from build123d import *

# Parameters (mm, degrees)
EXTRUDE1_DEPTH = 76.968
EXTRUDE2_DEPTH = 90
EXTRUDE3_DEPTH = 101.968
EXTRUDE4_DEPTH = 76.321
EXTRUDE5_DEPTH = 126.968
EXTRUDE6_DEPTH = 126.968
EXTRUDE7_DEPTH = 88.484


with BuildPart() as part:
    # Sketch1 → Extrude1 (new body)
    with BuildSketch(Plane(origin=(0, 0, 0), x_dir=(1, 0, 0), z_dir=(0, 1, 0))):
        Polygon((0, 0), (0, 55), (90, 77.5), (90, -22.5), align=None)
    extrude(amount=EXTRUDE1_DEPTH)

    # Sketch2 → Extrude2 (cut, symmetric)
    with BuildSketch(Plane.XY):
        Polygon((90, 76.968), (0, 35.000310766), (0, 76.968), align=None)
    extrude(amount=EXTRUDE2_DEPTH, both=True, mode=Mode.SUBTRACT)

    # Sketch3 → Extrude3 (add)
    with BuildSketch(Plane(origin=(0, 0, 0), x_dir=(1, 0, 0), z_dir=(0, 1, 0))):
        Polygon((90, 62.5), (20, 45), (20, 10), (90, -7.5), align=None)
    extrude(amount=EXTRUDE3_DEPTH)

    # Sketch4 → Extrude4 (cut, symmetric)
    with BuildSketch(Plane.XY):
        Polygon((90, 101.968), (20, 69.326463929), (20, 101.968), align=None)
    extrude(amount=EXTRUDE4_DEPTH, both=True, mode=Mode.SUBTRACT)

    # Sketch5 → Extrude5 (add)
    with BuildSketch(Plane(origin=(0, 0, 0), x_dir=(1, 0, 0), z_dir=(0, 1, 0))):
        Polygon((90, 47.5), (40, 35), (40, 20), (90, 7.5), align=None)
    extrude(amount=EXTRUDE5_DEPTH)

    # Sketch6 → Extrude6 (cut)
    with BuildSketch(Plane.XY):
        Polygon((90, 126.968), (40, 103.652617092), (40, 126.968), align=None)
    extrude(amount=-EXTRUDE6_DEPTH, mode=Mode.SUBTRACT)

    # Sketch7 → Extrude7 (cut, symmetric)
    with BuildSketch(Plane.XY):
        with BuildLine():
            Line((80, 0), (10, 0))
            ThreePointArc((10, 0), (45, 35), (80, 0))
        make_face()
    extrude(amount=EXTRUDE7_DEPTH, both=True, mode=Mode.SUBTRACT)


solid = part.part
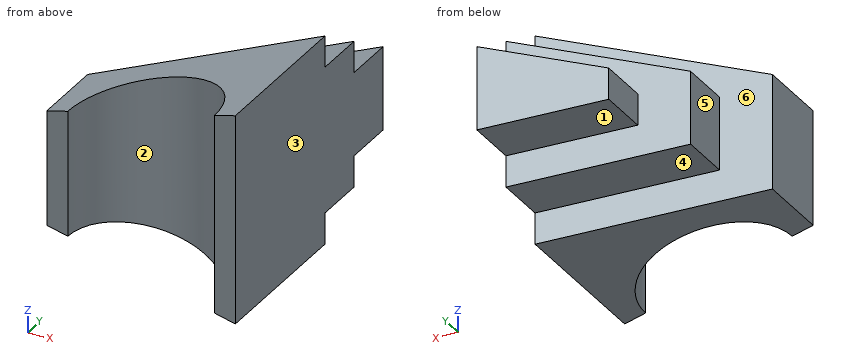
Check sheet for the modelled part. Datum: model origin and axes. Units: mm. Face numbers are marked on the shaded views. A direction names the side the tool comes from. Give positions to 0.01 mm unless a question says otherwise; leave off trailing zeros. Loops run counter-clockwise (first coordinate to the right, second up) from the corner with the lowest first, then second, coordinate; pieces in that order, holes last. Notation, with made-up numbers: M -5,4.25 L 24,4.25 A17 ccw 24,29.25 Z; hole C -24,66 d8. An arc over 180 degrees is marked long. Answer as a JSON object with one key per item and string values. Group by question number.
Q1. Cross-section at C-C on z = -5. Record the cut outline in (x, y), then the cut area to 3 significant figures.
Q2. Cross-section at D-D on y = 87. Record the cut outline in (x, z).
Q3. Release check for a two-part mould opening along X. For the marked faces 1, 2 and 3 record: released by +X, released by -X, zero draft, split by the parting line, or undercut.
Q4. Cross-section at B-B on x = 69. Record the cut outline in (y, z), then the cut area to 3 significant figures.
Q5. Go/stop test with flat-tipped pins: P1, Ø4, axis at y = 41, z = -12.5, coming from the -X side; P2, Ø1, axis at x = 50, z = -45, coming from the +Y side; P3, Ø6, axis at x = 16, z = -65, coming from the +Y side; P4, Ø2, axis at x = 80, y = 63.5, coming from the +Z side. Record where each tip stops, or that it passes through.
Q6. Cross-section at A-A on y = 10.5. Record the cut outline in (x, z), then the cut area to 3 significant figures.
Q7. Access from +Z, -Z, +X, -X, +Y, -Y to the whole of each face (thin tool, end or side, straight path). Record for the marked faces 4, 5 and 6.
Q8. Material ranges on line 1 along X through (y, z) = (95, -31.5); line 2 along Z through (x, y) = (42.5, 78) (3 decimals); line 3 along Y through (x, z) = (26.5, -7), recorded low to high. Write a range as [from, to].
Evaluation:
{
 "1": {"outline": "M 0,0 L 10,0 A35 cw 80,0 L 90,0 L 90,101.97 L 40,78.65 L 40,53.65 L 0,35 Z", "area": "4,360 mm2"},
 "2": {"outline": "M 40,-35 L 57.9,-39.48 L 57.9,-54.48 L 90,-62.5 L 90,7.5 L 57.9,-0.52 L 57.9,-15.52 L 40,-20 Z"},
 "3": {"face 1": "released by -X", "face 2": "undercut", "face 3": "released by +X"},
 "4": {"outline": "M 25.48,-72.25 L 67.18,-72.25 L 67.18,-57.25 L 92.18,-57.25 L 92.18,-42.25 L 117.18,-42.25 L 117.18,-12.75 L 92.18,-12.75 L 92.18,2.25 L 67.18,2.25 L 67.18,17.25 L 25.48,17.25 Z", "area": "5,960 mm2"},
 "5": {"P1": "stops at x = 8.58", "P2": "stops at y = 83.55", "P3": "passes through", "P4": "stops at z = 20.25"},
 "6": {"outline": "M 0,-55 L 11.61,-57.9 L 11.61,2.9 L 0,0 Z; M 78.39,-74.6 L 90,-77.5 L 90,22.5 L 78.39,19.6 Z", "area": "1,800 mm2"},
 "7": {"face 4": "-Z, -X, +Y", "face 5": "+Z, -Z, -X, +Y", "face 6": "-X, +Y"},
 "8": {"line 1": "x = [40, 90]", "line 2": "z = [-50.625, -4.375]", "line 3": "y = [29.71, 47.36]"}
}
